from build123d import *

# Parameters (mm, degrees)
F0_W     = 533.4
F0_H     = 609.6
F1_DEPTH = 31.75
F2_R     = 3.175
F3_R     = 40
F4_DEPTH = 31.751


with BuildPart() as f1:
    # F0 (on Top) → F1 (new body)
    with BuildSketch(Plane.XY):
        Rectangle(F0_W, F0_H)
    extrude(amount=F1_DEPTH)

    # F2
    f2_edges = [f1.edges().sort_by_distance(p)[0] for p in [
        (0, -304.8, 31.75),
        (-266.7, 0, 31.75),
        (266.7, 0, 31.75),
        (266.7, 0, 0),
        (0, -304.8, 0),
        (-266.7, 0, 0),
        (-266.7, -304.8, 15.875),
        (266.7, -304.8, 15.875),
    ]]
    fillet(f2_edges, radius=F2_R)

    # F3 (on face) → F4 (cut, through all)
    with BuildSketch(Plane.XY.offset(31.75)):
        with Locations((0, 209.55)):
            Circle(F3_R)
    extrude(amount=-F4_DEPTH, mode=Mode.SUBTRACT)


solid = f1.part
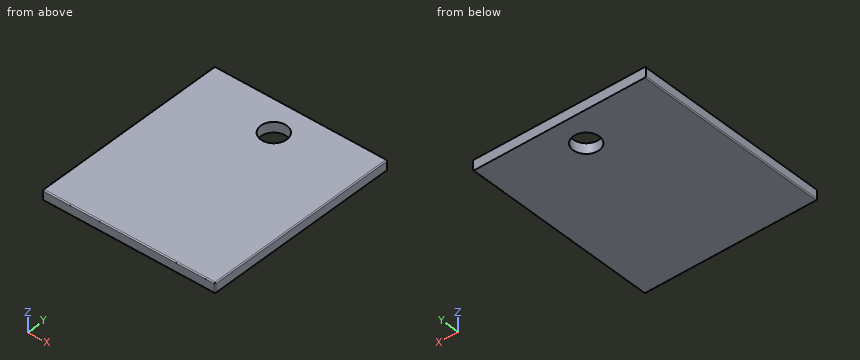
Verification items for the finished model (mm, model axes). Give positions to 0.01 mm unless a question says otherwise; leave off trailing zeros. Order: outer loops, then holes, each group sorted by start corner. A loop starts at its lowest first (then second) coordinate and runs counter-clockwise, first axis right, second up. Notation, with made-up numbers: M 36,9 L 82,9 A6 cw 82,14 Z; hole C 2.5,20 d7. An arc over 180 degrees is marked long. Answer as a JSON object with one key per item and string values. Group by question number.
1) Cross-section at C-C (z = 9). Enter the section's corners in (x, y) (3 decimals), then the cut area to 3 significant figures.
2) Scan lines: line 1 along Y through (x, z) = (0, 12); line 2 along X through (y, z) = (186.5, 2); line 3 along X through (y, z) = (127, 29). Record each from-to range of solid material in increasing order. Write a range as [from, to].
3) Cross-section at A-A (y = 209.55). Enter the section's corners in (x, z) (3 decimals).
4) Cross-section at B-B (x = 0). Enter the section's corners in (y, z) (3 decimals), then the cut area to 3 significant figures.
Result sheet:
{
 "1": {"outline": "M -266.7,-301.625 A3.175 ccw -263.525,-304.8 L 263.525,-304.8 A3.175 ccw 266.7,-301.625 L 266.7,304.8 L -266.7,304.8 Z; hole C 0,209.55 d80", "area": "320,000 mm2"},
 "2": {"line 1": "y = [-304.8, 169.55], [249.55, 304.8]", "line 2": "x = [-266.47, -32.69], [32.69, 266.47]", "line 3": "x = [-266.67, 266.67]"},
 "3": {"outline": "M -266.7,3.175 A3.175 ccw -263.525,0 L -40,0 L -40,31.75 L -263.525,31.75 A3.175 ccw -266.7,28.575 Z; M 40,0 L 263.525,0 A3.175 ccw 266.7,3.175 L 266.7,28.575 A3.175 ccw 263.525,31.75 L 40,31.75 Z"},
 "4": {"outline": "M -304.8,3.175 A3.175 ccw -301.625,0 L 169.55,0 L 169.55,31.75 L -301.625,31.75 A3.175 ccw -304.8,28.575 Z; M 249.55,0 L 304.8,0 L 304.8,31.75 L 249.55,31.75 Z", "area": "16,800 mm2"}
}
